Autodesk Inventor part; units mm, degrees
ref_plane "YZ Plane" through (0, 0, 0) normal (1, 0, 0) x (0, 1, 0)
ref_plane "XZ Plane" through (0, 0, 0) normal (0, 1, 0) x (-1, 0, 0)
ref_plane "XY Plane" through (0, 0, 0) normal (0, 0, 1) x (1, 0, 0)
sketch "Sketch1" plane through (0, 0, 0) normal (0, 1, 0) x (-1, 0, 0)
  line L0 (0, -23.07) -> (-48.1, -23.07)
  line L1 (-48.1, -23.07) -> (-48.1, 0)
  line L2 (-48.1, 0) -> (0, 0)
  line L3 (0, 0) -> (0, -23.07)
  point P0 (0, 0)
  dimension "d0" = 48.1
  dimension "d1" = 23.07
extrude "Extrusion1" add sketch "Sketch1" along normal blind 1.6
sketch "Sketch2" plane through (0, 1.6, 0) normal (0, 1, 0) x (1, 0, 0)
  line L0 (33.6, 23.07) -> (43.1, 23.07)
  line L1 (43.1, 23.07) -> (43.1, 18.57)
  line L2 (43.1, 18.57) -> (33.6, 18.57)
  line L3 (33.6, 18.57) -> (33.6, 23.07)
  line L4 (48.1, 23.07) -> (0, 23.07)
  line L5 (48.1, 0) -> (48.1, 23.07)
  line L6 (23.6, 23.07) -> (33.1, 23.07)
  line L7 (33.1, 23.07) -> (33.1, 18.57)
  line L8 (33.1, 18.57) -> (23.6, 18.57)
  line L9 (23.6, 18.57) -> (23.6, 23.07)
  line L10 (13.6, 23.07) -> (23.1, 23.07)
  line L11 (23.1, 23.07) -> (23.1, 18.57)
  line L12 (23.1, 18.57) -> (13.6, 18.57)
  line L13 (13.6, 18.57) -> (13.6, 23.07)
  point P0 (0, 0)
  dimension "d4" = 9.5
  dimension "d5" = 4.5
  dimension "d6" = 5
  dimension "d7" = 9.5
  dimension "d8" = 4.5
  dimension "d9" = 0.5
  dimension "d10" = 9.5
  dimension "d11" = 4.5
  dimension "d12" = 0.5
extrude "Extrusion2" add sketch "Sketch2" along normal blind 10
sketch "Sketch3" plane through (0, 1.6, 0) normal (0, 1, 0) x (1, 0, 0)
  line L0 (48.1, 0) -> (48.1, 23.07)
  line L1 (48.1, 23.07) -> (45.1, 23.07)
  line L2 (45.1, 23.07) -> (45.1, 20.07)
  line L3 (45.1, 20.07) -> (48.1, 20.07)
  line L4 (48.1, 20.07) -> (48.1, 23.07)
  line L5 (0, 23.07) -> (3, 23.07)
  line L6 (3, 23.07) -> (3, 20.07)
  line L7 (3, 20.07) -> (0, 20.07)
  line L8 (0, 20.07) -> (0, 23.07)
  line L9 (0, 0) -> (3, 0)
  line L10 (3, 0) -> (3, 3)
  line L11 (3, 3) -> (0, 3)
  line L12 (0, 3) -> (0, 0)
  line L13 (48.1, 0) -> (45.1, 0)
  line L14 (45.1, 0) -> (45.1, 3)
  line L15 (45.1, 3) -> (48.1, 3)
  line L16 (48.1, 3) -> (48.1, 0)
  dimension "d15" = 3
  dimension "d16" = 3
  dimension "d17" = 3
extrude "Extrusion3" add sketch "Sketch3" along normal blind 10
sketch "Sketch4" plane through (0, 1.6, 0) normal (0, 1, 0) x (1, 0, 0)
  circle A0 centre (39.1, 4) radius 4
  line L0 (48.1, 3) -> (48.1, 20.07)
  circle A1 centre (4, 11) radius 4
  point P0 (0, 0)
  dimension "d20" = 8
  dimension "d21" = 9
  dimension "d22" = 8
extrude "Extrusion4" add sketch "Sketch4" along normal blind 11
sketch "Sketch5" plane through (0, 1.6, 0) normal (0, 1, 0) x (1, 0, 0)
  line L0 (21.9, 12.1) -> (33.9, 12.1)
  line L1 (33.9, 12.1) -> (33.9, 0)
  line L2 (33.9, 0) -> (21.9, 0)
  line L3 (21.9, 0) -> (21.9, 12.1)
  circle A0 centre (39.1, 4) radius 4
  point P0 (0, 0)
  dimension "d25" = 12
  dimension "d26" = 12.1
  dimension "d27" = 1.2
extrude "Extrusion5" add sketch "Sketch5" along normal blind 6 contours L0 L1 L2 L3
properties part number "LM2596 Buck Converter"
Design review of the part built by this model. Coordinates are the model's own, in mm. A direction names the side the tool comes from. Give positions to 0.01 mm unless a question says otherwise; leave off trailing zeros. Order: outer loops, then holes, each group sorted by start corner. A loop starts at its lowest first (then second) coordinate and runs counter-clockwise, first axis right, second up. Notation, with made-up numbers: M 58,-29.5 L 102,-29.5 A29 ccw 102,-7.5 Z; hole C 2.25,66.25 d4. An arc over 180 degrees is marked long. One line per question, with ' | ' between items. Start each with the question number.
Q1. We need section C-C (x = 27). Write out the cut boundary in (y, z), plus the area to 3 significant figures.
Q2. For L1, parallel to X at y = 4.25, z = -21.25; L2, parallel to Z at x = 22, y = 5.75; L3, parallel to Z at x = 33, y = 10.75, list the stretches that pass through material, from the lowest coordinate up. Write a range as [from, to].
Q3. The part is to be moulded in two halves that separate along X. For faces 4 (the face through (24, 1.6, -14)), 5 (the face through (1, 11.6, -22)), 6 (the face through (0, 1, -11)), say which applies: +X half, -X half, draft (parallel to the pull), parting line (faces both ways), or undercut.
Q4. We need section D-D (z = -4). Write out the cut boundary in (x, y).
Q5. We need section A-A (y = 2.75). State how many separate pieces and enclosed holes the cut face has, plus the area to 3 significant figures.
Q6. For pin 1 Ø3.5 at (x, z) = (1, -1.5) entering from +Y; pin 2 Ø1 at (x, z) = (12.5, -4) entering from +Y; pin 3 Ø5 at (x, y) = (20.5, 8.5) entering from +Z; pin 4 Ø4 at (y, z) = (4, -6) entering from -X, all flat-tipped, find the tip position at first contact; note any pin that passes through.
Q7. Machinability: for faces 1 (the face through (38, 11.6, -21)), 2 (the face through (23.6, 7, -21)), 3 (the face through (2, 7, -3)), which of the approach directions +Z, -Z, +X, -X, +Y, -Y give a long, thin tool a straight path to every point of the face, cutting with its end or side? Answer none if there is none.
Returned:
1) outline: M 0,-23.07 L 11.6,-23.07 L 11.6,-18.57 L 1.6,-18.57 L 1.6,-12.1 L 7.6,-12.1 L 7.6,0 L 0,0 Z | area: 155 mm2
2) L1: [0, 3], [13.6, 23.1], [23.6, 33.1], [33.6, 43.1], [45.1, 48.1] | L2: [-23.07, -18.57], [-12.1, 0] | L3: [-23.07, -18.57]
3) face 4: undercut | face 5: draft | face 6: -X half
4) outline: M 0,0 L 48.1,0 L 48.1,1.6 L 43.1,1.6 L 43.1,12.6 L 35.1,12.6 L 35.1,1.6 L 33.9,1.6 L 33.9,7.6 L 21.9,7.6 L 21.9,1.6 L 0,1.6 Z
5) separate pieces: 10 | enclosed holes: 0 | area: 410 mm2
6) pin 1: y = 11.6 | pin 2: y = 1.6 | pin 3: z = 0 | pin 4: x = 1.35
7) face 1: -Z, +X, -X, +Y | face 2: -Z, +Y | face 3: -X, +Y
